Model file for the job. Use its own axes, mm. Face numbers are marked on the shaded views. A direction names the side the tool comes from. Coordinates: 2 decimals unless noted, no trailing zeros. Order: outer loops, then holes, each group sorted by start corner. A loop starts at its lowest first (then second) coordinate and runs counter-clockwise, first axis right, second up. Notation, with made-up numbers: (28, 23) -> (82, 23) arc R18 ccw to (82, 50) -> close; hole circle Ø8 at (-21, -20). An arc over 180 degrees is marked (long way). Return JSON: item names as keys, results as strings. Group by question number.
1) Which spindle directions (+Z, -Z, +X, -X, +Y, -Y) get a long thin tool onto all of the face, cutting with end or side? Do the marked faces 1, 2, 3, 4 and 5. Say none if no direction does.
2) Cut at B-B (y = 57.5). Write the cut outline in (x, z).
3) Cut at C-C (x = 13). Write the cut outline in (y, z).
4) Cut at A-A (z = -22.5). Write the cut outline in (x, y).
5) Probe line 1 (Z direction, x = -8, y = 5); line 2 (X direction, y = 20.5, z = 1.5); line 3 (Z direction, x = 47.5, y = 56.5). List the from-to ranges inside material, lowest first.
6) Flat gauge pins, fed straight in: pin 1 (0.9 mm diameter, centred on x = 39.5, z = 27.5, fed in from +Y); pin 2 (3 mm diameter, centred on y = 6.5, z = -22.5, fed in from -X); pin 3 (22 mm diameter, centred on y = 26, z = 10, fed in from -X); pin 4 (1 mm diameter, centred on x = -10.5, z = -4.5, fed in from -Y). Where does each tip first touch, or does it go through?
7) Pull direction Z, two halves, no side cores. Call the marked faces 6, 7, 8 and 9: +Z half, -Z half, draft (parallel to the pull), parting line (faces both ways), or undercut.
8) Cut at D-D (z = -6.5). Write the cut outline in (x, y).
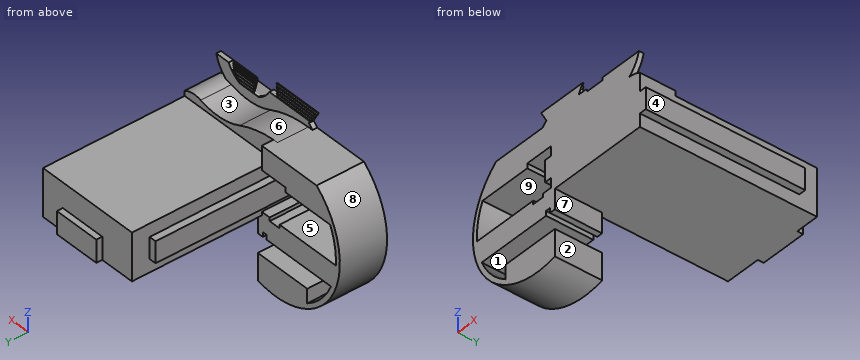
from build123d import *

# Parameters (mm, degrees)
EXTRUDE_1_DEPTH          = 20
EXTRUDE_2_DEPTH          = 75
CUT_EXTRUDE_1_REACH      = 104.675
SKETCH_4_W               = 3
SKETCH_4_H               = 7.5
CUT_EXTRUDE_3_DEPTH      = 15
SKETCH_10_W              = 45
SKETCH_10_H              = 8.5
CUT_EXTRUDE_4_DEPTH      = 5
EXTRUDE_7_DEPTH          = 2
CUT_EXTRUDE_5_REACH      = 99.006
CUT_EXTRUDE_6_DEPTH      = 21
CUT_EXTRUDE_7_REACH      = 99.006
SKETCH_16_R              = 11.5
EXTRUDE_8_DEPTH          = 11
EXTRUDE_8_DEPTH_BACK     = 11
CUT_EXTRUDE_8_REACH      = 106.745
CUT_EXTRUDE_8_END_RADIUS = 11.5
SKETCH_22_W              = 20
SKETCH_22_H              = 9.5
EXTRUDE_9_DEPTH          = 2.5


with BuildPart() as part:
    # 草图1 → 凸台-拉伸1 (new body)
    with BuildSketch(Plane(origin=(0, 0, 0), x_dir=(1, 0, 0), z_dir=(0, 1, 0))):
        with BuildLine():
            Line((-20.766559657, -25), (52, -25))
            Line((52, -25), (52, -15))
            Line((52, -15), (-5, -15))
            Line((-5, -15), (-5, -13))
            Line((-5, -13), (-27.590759323, -13))
            ThreePointArc((-27.590759323, -13), (-29.966289228, -5.680801874), (-30.434355587, 2))
            Line((-30.434355587, 2), (-2, 2))
            Line((-2, 2), (-2, 3.5))
            Line((-2, 3.5), (3, 3.5))
            Line((3, 3.5), (3, 2))
            Line((3, 2), (9, 2))
            Line((9, 2), (9, 12))
            Line((9, 12), (6.5, 12))
            Line((6.5, 12), (6.5, 10))
            Line((6.5, 10), (4.5, 10))
            Line((4.5, 10), (4.5, 12))
            Line((4.5, 12), (-28.040149786, 12))
            ThreePointArc((-28.040149786, 12), (-23.100827955, 19.914862485), (-16, 25.966324345))
            Line((-16, 25.966324345), (-16, 20))
            Line((-16, 20), (9, 20))
            Line((9, 20), (9, 31.228992939))
            ThreePointArc((9, 31.228992939), (-28.723472863, 15.205660351), (-20.766559657, -25))
        make_face()
    extrude(amount=EXTRUDE_1_DEPTH)

    # 草图3 → 凸台-拉伸2 (add)
    with BuildSketch(Plane(origin=(0, 0, 0), x_dir=(1, 0, 0), z_dir=(0, 1, 0))):
        Polygon((7, 3.5), (52, 3.5), (52, -2), (55, -2), (55, -11), (52, -11), (52, -16.5), (7, -16.5), (7, -11), (4, -11), (4, -2), (7, -2), align=None)
    extrude(amount=EXTRUDE_2_DEPTH)

    # 草图4 → 切除-拉伸1 (cut, up to next)
    with BuildSketch(Plane.XY.offset(11), mode=Mode.PRIVATE) as cut_extrude_1_sk1:
        with Locations((5.5, 71.25)):
            Rectangle(SKETCH_4_W, SKETCH_4_H)
    cut_extrude_1_tool1 = extrude(cut_extrude_1_sk1.sketch, amount=-CUT_EXTRUDE_1_REACH, mode=Mode.PRIVATE) & part.part
    # 草图4 → 切除-拉伸1 (cut, up to next)
    with BuildSketch(Plane.XY.offset(11), mode=Mode.PRIVATE) as cut_extrude_1_sk2:
        with Locations((53.5, 71.25)):
            Rectangle(SKETCH_4_W, SKETCH_4_H)
    cut_extrude_1_tool2 = extrude(cut_extrude_1_sk2.sketch, amount=-CUT_EXTRUDE_1_REACH, mode=Mode.PRIVATE) & part.part
    add(cut_extrude_1_tool1.solids().sort_by_distance((5.5, 71.25, 11))[0], mode=Mode.SUBTRACT)
    add(cut_extrude_1_tool2.solids().sort_by_distance((53.5, 71.25, 11))[0], mode=Mode.SUBTRACT)

    # 草图9 → 切除-拉伸3 (cut)
    with BuildSketch(Plane(origin=(0, 0, 0), x_dir=(1, 0, 0), z_dir=(0, 1, 0))):
        with BuildLine():
            Line((52, -25), (52, -18.660254038))
            ThreePointArc((52, -18.660254038), (48.035984141, -19.946192078), (43.892048311, -19.504769134))
            ThreePointArc((43.892048311, -19.504769134), (33.901437956, -18.227421286), (24.144020863, -20.724764765))
            ThreePointArc((24.144020863, -20.724764765), (14.807792452, -23.918187659), (5, -25))
            Line((5, -25), (52, -25))
        make_face()
    extrude(amount=CUT_EXTRUDE_3_DEPTH, mode=Mode.SUBTRACT)

    # 草图10 → 切除-拉伸4 (cut)
    with BuildSketch(Plane(origin=(0, 20, 0), x_dir=(1, 0, 0), z_dir=(0, 1, 0))):
        with Locations((29.5, -20.75)):
            Rectangle(SKETCH_10_W, SKETCH_10_H)
    extrude(amount=-CUT_EXTRUDE_4_DEPTH, mode=Mode.SUBTRACT)

    # 草图11 → 凸台-拉伸7 (add)
    with BuildSketch(Plane(origin=(0, 0, 0), x_dir=(1, 0, 0), z_dir=(0, 1, 0))):
        with BuildLine():
            Line((2, -31.5), (4.744300512, -26.75984457))
            ThreePointArc((4.744300512, -26.75984457), (2.188260872, -20.573315931), (7.5, -16.5))
            Line((7.5, -16.5), (37, -16.5))
            ThreePointArc((37, -16.5), (47.606601718, -20.893398282), (52, -31.5))
            Line((52, -31.5), (2, -31.5))
        make_face()
    extrude(amount=EXTRUDE_7_DEPTH)

    # 草图13 → 切除-拉伸5 (cut, up to next)
    with BuildSketch(Plane(origin=(0, 2, 0), x_dir=(1, 0, 0), z_dir=(0, 1, 0)), mode=Mode.PRIVATE) as cut_extrude_5_sk1:
        Polygon((22.995595677, -31.5), (20.996905673, -27.799311895), (54.018038791, -27.799311895), (54.018038791, -31.5), align=None)
    cut_extrude_5_tool1 = extrude(cut_extrude_5_sk1.sketch, amount=-CUT_EXTRUDE_5_REACH, mode=Mode.PRIVATE) & part.part
    add(cut_extrude_5_tool1.solids().sort_by_distance((38.001947, 2, 29.630407))[0], mode=Mode.SUBTRACT)

    # 草图15 → 切除-拉伸6 (cut)
    with BuildSketch(Plane(origin=(2, 0, 0), x_dir=(0, 0, -1), z_dir=(1, 0, 0))):
        Polygon((-31.5, 0.4), (-30.574311895, 0.4), (-30.574311895, 0.8), (-29.649311895, 0.8), (-29.649311895, 1.2), (-28.724311895, 1.2), (-28.724311895, 1.6), (-27.799311895, 1.6), (-27.799311895, 2), (-31.5, 2), align=None)
    extrude(amount=CUT_EXTRUDE_6_DEPTH, mode=Mode.SUBTRACT)

    # 草图16 → 切除-拉伸7 (cut, up to next)
    with BuildSketch(Plane(origin=(0, 2, 0), x_dir=(1, 0, 0), z_dir=(0, 1, 0)), mode=Mode.PRIVATE) as cut_extrude_7_sk1:
        with Locations((35, -33)):
            Circle(SKETCH_16_R)
    cut_extrude_7_tool1 = extrude(cut_extrude_7_sk1.sketch, amount=-CUT_EXTRUDE_7_REACH, mode=Mode.PRIVATE) & part.part
    add(cut_extrude_7_tool1.solids().sort_by_distance((35, 2, 33))[0], mode=Mode.SUBTRACT)

    # 草图18 → 凸台-拉伸8 (add, two sides: drawn at the far end of the back side and taken through both)
    with BuildSketch(Plane(origin=(35, 0, 0), x_dir=(0, 0, -1), z_dir=(1, 0, 0)).offset(-EXTRUDE_8_DEPTH_BACK)):
        Polygon((-27.799311895, 0.25), (-27.799311895, 0), (-21.5, 0), (-21.5, 2), (-22.5, 2), (-22.5, 1.75), (-23.5, 1.75), (-23.5, 1.5), (-24.5, 1.5), (-24.5, 1.25), (-25.5, 1.25), (-25.5, 1), (-26, 1), (-26, 0.75), (-26.5, 0.75), (-26.5, 0.5), (-27, 0.5), (-27, 0.25), align=None)
    extrude(amount=EXTRUDE_8_DEPTH + EXTRUDE_8_DEPTH_BACK)

    # 切除-拉伸8: up to this cylinder (the profile starts inside it)
    cut_extrude_8_end = Plane(origin=(35, 1.199158, 33), z_dir=(0, 1, 0)) * Cylinder(CUT_EXTRUDE_8_END_RADIUS, 237.49, mode=Mode.PRIVATE)
    # 草图21 → 切除-拉伸8 (cut, up to the surface)
    with BuildSketch(Plane(origin=(33, 0, 0), x_dir=(0, 0, -1), z_dir=(1, 0, 0)), mode=Mode.PRIVATE) as cut_extrude_8_sk1:
        with BuildLine():
            Line((-22.5, 2), (-27.799311895, 2.043691233))
            Line((-27.799311895, 2.043691233), (-27.799311895, 0))
            add(Edge.make_bspline(
                [(-27.799311895, 0), (-27.204791672, -0.222081078), (-26.384663507, 0.078646126), (-25.326854987, 0.456459594), (-24.66401125, 0.700176127), (-24.021132133, 0.799941058), (-23.26371078, 1.202357465), (-22.499729223, 1.183276831), (-22.5, 2)],
                knots=[0, 0, 0, 0, 0.297814847, 0.424941071, 0.570246023, 0.652881605, 0.750360442, 1, 1, 1, 1], degree=3))
        make_face()
    cut_extrude_8_tool1 = extrude(cut_extrude_8_sk1.sketch, amount=-CUT_EXTRUDE_8_REACH, mode=Mode.PRIVATE) & cut_extrude_8_end
    add(cut_extrude_8_tool1.solids().sort_by_distance((33, 1.199158, 25.64967))[0], mode=Mode.SUBTRACT)

    # 草图22 → 凸台-拉伸9 (add)
    with BuildSketch(Plane(origin=(0, 75, 0), x_dir=(1, 0, 0), z_dir=(0, 1, 0))):
        with Locations((32, -1.25)):
            Rectangle(SKETCH_22_W, SKETCH_22_H)
    extrude(amount=EXTRUDE_9_DEPTH)


solid = part.part
Answers below:
{
 "1": {"face 1": "+X, +Y, -Y", "face 2": "-Z, +X, +Y, -Y", "face 3": "+Z, +Y", "face 4": "+Z, -Z, +X, +Y, -Y", "face 5": "+Y, -Y"},
 "2": {"outline": "(4, 2) -> (7, 2) -> (7, -3.5) -> (52, -3.5) -> (52, 2) -> (55, 2) -> (55, 11) -> (52, 11) -> (52, 16.5) -> (7, 16.5) -> (7, 11) -> (4, 11) -> close"},
 "3": {"outline": "(0, -3.5) -> (75, -3.5) -> (75, 16.5) -> (15, 16.5) -> (15, 24.28) -> (2, 24.28) -> (2, 27.8) -> (1.6, 27.8) -> (1.6, 28.72) -> (1.2, 28.72) -> (1.2, 29.65) -> (0.8, 29.65) -> (0.8, 30.57) -> (0.4, 30.57) -> (0.4, 31.5) -> (0, 31.5) -> close"},
 "4": {"outline": "(-23.45, 0) -> (-20.59, 0) -> (-20.59, 20) -> (-23.45, 20) -> close; (-16, 0) -> (9, 0) -> (9, 20) -> (-16, 20) -> close"},
 "5": {"line 1": "z = -31.5 to -20, -12 to -2, 13 to 25", "line 2": "x = 7 to 52", "line 3": "z = -3.5 to 16.5"},
 "6": {"pin 1": "stops at y = 0.25", "pin 2": "stops at x = -24.8", "pin 3": "stops at x = -32.49", "pin 4": "stops at y = 0"},
 "7": {"face 6": "+Z half", "face 7": "draft", "face 8": "parting line", "face 9": "undercut"},
 "8": {"outline": "(-31.84, 0) -> (9, 0) -> (9, 20) -> (-31.84, 20) -> close"}
}
